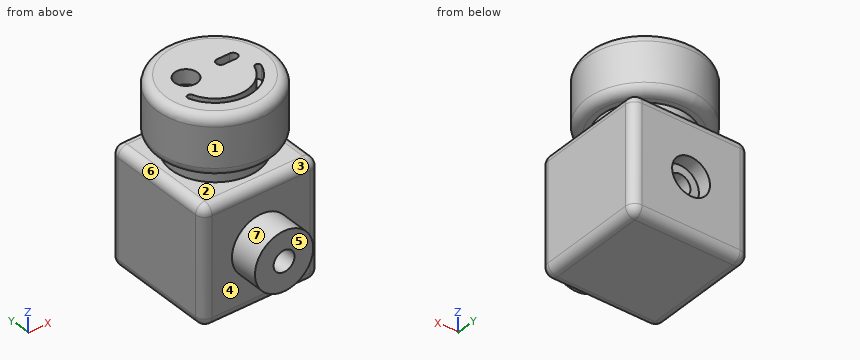
from build123d import *

# Parameters (mm, degrees)
SKETCH1_R                                            = 5
BOSS_EXTRUDE1_DEPTH                                  = 5
SKETCH2_W                                            = 20
SKETCH2_H                                            = 20
BOSS_EXTRUDE2_DEPTH                                  = 20
SKETCH3_R                                            = 7.5
BOSS_EXTRUDE4_DEPTH                                  = 2.5
SKETCH4_R                                            = 10
BOSS_EXTRUDE5_DEPTH                                  = 10
CBORE_FOR_M3_HEX_SOCKET_THIN_HEAD_CAP_SC_D           = 3.6
CBORE_FOR_M3_HEX_SOCKET_THIN_HEAD_CAP_SC_CBORE_D     = 6.5
CBORE_FOR_M3_HEX_SOCKET_THIN_HEAD_CAP_SC_CBORE_DEPTH = 2.4
FILLET1_R                                            = 1.5875
SKETCH7_R                                            = 1.948257307
CUT_EXTRUDE2_DEPTH                                   = 2.5


with BuildPart() as part:
    # Sketch1 → Boss-Extrude1 (new body)
    with BuildSketch(Plane(origin=(0, 0, 0), x_dir=(1, 0, 0), z_dir=(0, 1, 0))):
        with Locations(Location((0, 0, 0), (0, 0, 270))):
            Circle(SKETCH1_R)
    extrude(amount=BOSS_EXTRUDE1_DEPTH)

    # Sketch2 → Boss-Extrude2 (add)
    with BuildSketch(Plane(origin=(0, 5, 0), x_dir=(1, 0, 0), z_dir=(0, 1, 0))):
        Rectangle(SKETCH2_W, SKETCH2_H)
    extrude(amount=BOSS_EXTRUDE2_DEPTH)

    # Sketch3 → Boss-Extrude4 (add)
    with BuildSketch(Plane.XY.offset(10)):
        with Locations((0, 15)):
            Circle(SKETCH3_R)
    extrude(amount=BOSS_EXTRUDE4_DEPTH)

    # Sketch4 → Boss-Extrude5 (add)
    with BuildSketch(Plane.XY.offset(12.5)):
        with Locations((0, 15)):
            Circle(SKETCH4_R)
    extrude(amount=BOSS_EXTRUDE5_DEPTH)

    # CBORE for M3 Hex Socket Thin Head Cap Screw1 (through all)
    with Locations(Plane(origin=(0, 25, 0), x_dir=(1, 0, 0), z_dir=(0, 1, 0))):
        with Locations((0, 0)):
            CounterBoreHole(CBORE_FOR_M3_HEX_SOCKET_THIN_HEAD_CAP_SC_D / 2, CBORE_FOR_M3_HEX_SOCKET_THIN_HEAD_CAP_SC_CBORE_D / 2, CBORE_FOR_M3_HEX_SOCKET_THIN_HEAD_CAP_SC_CBORE_DEPTH)

    # Fillet1
    fillet1_edges = [part.edges().sort_by_distance(p)[0] for p in [
        (-10, 15, 12.5),
        (-10, 15, 22.5),
        (10, 5, 0),
        (10, 15, 10),
        (0, 5, -10),
        (10, 15, -10),
        (-10, 5, 0),
        (-10, 15, -10),
        (0, 5, 10),
        (-10, 15, 10),
        (10, 25, 0),
        (0, 25, -10),
        (-10, 25, 0),
        (0, 25, 10),
    ]]
    fillet(fillet1_edges, radius=FILLET1_R)

    # Sketch7 → Cut-Extrude2 (cut)
    with BuildSketch(Plane.XY.offset(22.5)):
        with Locations((-3.508388237, 16.85452893)):
            Circle(SKETCH7_R)
        with BuildLine():
            Line((2.435234188, 17.597481733), (4.581542286, 17.597481733))
            ThreePointArc((4.581542286, 17.597481733), (5.32449509, 16.85452893), (4.581542286, 16.111576127))
            Line((4.581542286, 16.111576127), (2.435234188, 16.111576127))
            ThreePointArc((2.435234188, 16.111576127), (1.692281385, 16.85452893), (2.435234188, 17.597481733))
        make_face()
        with BuildLine():
            ThreePointArc((-6.253186094, 12.871476402), (-0.060422297, 8.394752224), (6.213201069, 12.757438628))
            ThreePointArc((6.213201069, 12.757438628), (5.912646592, 13.397490974), (5.272594245, 13.096936498))
            ThreePointArc((5.272594245, 13.096936498), (-0.05127506, 9.394710388), (-5.306526, 13.193710271))
            ThreePointArc((-5.306526, 13.193710271), (-5.940972981, 13.505923383), (-6.253186094, 12.871476402))
        make_face()
    extrude(amount=-CUT_EXTRUDE2_DEPTH, mode=Mode.SUBTRACT)


solid = part.part
CAD build for the part. Positions are in the model's coordinates, mm. Face numbers are marked on the shaded views. A direction names the side the tool comes from. Coordinates: 2 decimals unless noted, no trailing zeros. Loops run counter-clockwise (first coordinate to the right, second up) from the corner with the lowest first, then second, coordinate; pieces in that order, holes last. Notation, with made-up numbers: (78.25, 59.25) - (124.25, 59.25) arc R25 cw to (124.25, 89.25) - close; hole circle Ø4 at (4.5, -9.5). An arc over 180 degrees is marked (long way). Use one line per item in the form item = value. Start each with the question number.
1) Band-saw the part on B-B (y = 23). State how many separate pieces and enclosed holes the cut face has, and give its area (3 significant figures).
2) Drill centre lines: L1, parallel to Z at x = 0, y = 24.25; L2, parallel to X at y = 9.25, z = 8.5; L3, parallel to Z at x = 7.5, y = 9.25. Where is each one in solid material? Low to high. Write a range as from..to.
3) Tool access for the marked faces 1, 2, 3 and 4: list every direction of +Z, -Z, +X, -X, +Y, -Y with a clear straight run to the whole face (end or side of a thin tool).
4) Two-plate mould, pull along Z, no slides. Class the marked faces 5, 6 and 7: +Z half, -Z half, draft (parallel to the pull), parting line (faces both ways), or undercut.
5) Flat gauge pins, fed straight in: pin 1 (5 mm diameter, centred on x = -3.51, y = 16.85, fed in from +Z); pin 2 (0.6 mm diameter, centred on x = 3, z = 21, fed in from -Y); pin 3 (0.7 mm diameter, centred on x = 2.5, y = 17, fed in from +Z); pin 4 (8 mm diameter, centred on y = 22.5, z = 19, fed in from -X). Where does each tip first touch, or does it go through?
6) Band-saw the part on C-C (z = 12). Give the cut face in (x, y), and give its area (3 significant figures).
Check values:
q1.separate_pieces = 2
q1.enclosed_holes = 1
q1.area = 481 mm2
q2.L1 = -9.76..-3.25, 3.25..9.76, 12.74..22.26
q2.L2 = -10..10
q2.L3 = -10..10, 12.89..22.11
q3.face_1 = +Z
q3.face_2 = none
q3.face_3 = +X, -X, -Y
q3.face_4 = -Y
q4.face_5 = draft
q4.face_6 = undercut
q4.face_7 = parting line
q5.pin_1 = 22.5
q5.pin_2 = 5.37
q5.pin_3 = 20
q5.pin_4 = -9.37
q6.outline = circle Ø15 at (0, 15)
q6.area = 177 mm2
